Build history of the part. All positions in model axes, mm. A direction names the side the tool comes from. Coordinates: 2 decimals unless noted, no trailing zeros. Write each loop counter-clockwise with the first axis right and the second up, starting at its lowest first coordinate (ties: lowest second). Pieces come first, ordered by that corner, then holes.
```python
from build123d import *

# Parameters (mm, degrees)
SKETCH_1_W          = 37
SKETCH_1_H          = 37
EXTRUDE_1_DEPTH     = 11
SKETCH_2_R          = 1.5
CUT_EXTRUDE_1_DEPTH = 4
SKETCH_3_R          = 5.5
CUT_EXTRUDE_2_DEPTH = 29.381331893
SKETCH_4_R          = 7.5
CUT_EXTRUDE_4_DEPTH = 8
SKETCH_5_R          = 0.75
CUT_EXTRUDE_5_DEPTH = 28.358728041
SKETCH_7_W          = 8.873163899
SKETCH_7_H          = 2
SKETCH_7_W_2        = 8.897226177
SKETCH_7_W_3        = 2
SKETCH_7_H_2        = 11.172985464
EXTRUDE_3_DEPTH     = 5
EXTRUDE_6_DEPTH     = 8
EXTRUDE_7_REACH     = 44.805
EXTRUDE_8_REACH     = 44.805
CHAMFER_2_SIZE      = 3
SKETCH_11_R         = 0.75
CUT_EXTRUDE_6_DEPTH = 28.358728041
CHAMFER_3_SIZE      = 3
CHAMFER_3_SIZE2     = 4
FILLET_1_R          = 1
FILLET_2_R          = 1


with BuildPart() as part:
    # 草图1 → 凸台-拉伸1 (new body)
    with BuildSketch(Plane(origin=(0, 0, 0), x_dir=(1, 0, 0), z_dir=(0, 1, 0))):
        Rectangle(SKETCH_1_W, SKETCH_1_H)
    extrude(amount=EXTRUDE_1_DEPTH)

    # 草图2 → 切除-拉伸1 (cut)
    with BuildSketch(Plane.XZ):
        with Locations(Location((-16, 16, 0), (0, 0, 270))):
            Circle(SKETCH_2_R)
        with Locations(Location((-16, -16, 0), (0, 0, 270))):
            Circle(SKETCH_2_R)
        with Locations(Location((16, 16, 0), (0, 0, 270))):
            Circle(SKETCH_2_R)
        with Locations(Location((16, -16, 0), (0, 0, 270))):
            Circle(SKETCH_2_R)
        with Locations(Location((16, 4, 0), (0, 0, 270))):
            Circle(SKETCH_2_R)
        with Locations(Location((-16, 4, 0), (0, 0, 270))):
            Circle(SKETCH_2_R)
        with Locations(Location((0, 16, 0), (0, 0, 270))):
            Circle(SKETCH_2_R)
    extrude(amount=-CUT_EXTRUDE_1_DEPTH, mode=Mode.SUBTRACT)

    # 草图3 → 切除-拉伸2 (cut, through all)
    with BuildSketch(Plane.XZ):
        with Locations(Location((0, 0, 0), (0, 0, 270))):
            Circle(SKETCH_3_R)
    extrude(amount=-CUT_EXTRUDE_2_DEPTH, mode=Mode.SUBTRACT)

    # 草图4 → 切除-拉伸4 (cut)
    with BuildSketch(Plane.XZ):
        with BuildLine():
            Line((-16.5, 0.535898385), (-16.5, -12.535898385))
            ThreePointArc((-16.5, -12.535898385), (-13.525126266, -13.525126266), (-12.535898385, -16.5))
            Line((-12.535898385, -16.5), (12.535898385, -16.5))
            ThreePointArc((12.535898385, -16.5), (13.525126266, -13.525126266), (16.5, -12.535898385))
            Line((16.5, -12.535898385), (16.5, 0.535898385))
            ThreePointArc((16.5, 0.535898385), (12.5, 4), (16.5, 7.464101615))
            Line((16.5, 7.464101615), (16.5, 12.535898385))
            ThreePointArc((16.5, 12.535898385), (13.525126266, 13.525126266), (12.535898385, 16.5))
            Line((12.535898385, 16.5), (3.464101615, 16.5))
            ThreePointArc((3.464101615, 16.5), (0, 12.5), (-3.464101615, 16.5))
            Line((-3.464101615, 16.5), (-12.535898385, 16.5))
            ThreePointArc((-12.535898385, 16.5), (-13.525126266, 13.525126266), (-16.5, 12.535898385))
            Line((-16.5, 12.535898385), (-16.5, 7.464101615))
            ThreePointArc((-16.5, 7.464101615), (-12.5, 4), (-16.5, 0.535898385))
        make_face()
        with Locations(Location((0, 0, 0), (0, 0, 270))):
            Circle(SKETCH_4_R, mode=Mode.SUBTRACT)
    extrude(amount=-CUT_EXTRUDE_4_DEPTH, mode=Mode.SUBTRACT)

    # 草图5 → 切除-拉伸5 (cut, through all)
    with BuildSketch(Plane.XZ.offset(-8)):
        with Locations(Location((-8, 14, 0), (0, 0, 270))):
            Circle(SKETCH_5_R)
        with Locations(Location((0, 10.5, 0), (0, 0, 270))):
            Circle(SKETCH_5_R)
        with Locations(Location((8, 14, 0), (0, 0, 270))):
            Circle(SKETCH_5_R)
    extrude(amount=-CUT_EXTRUDE_5_DEPTH, mode=Mode.SUBTRACT)

    # 草图7 → 凸台-拉伸3 (add)
    with BuildSketch(Plane.XZ.offset(-8)):
        with Locations((-9.263191889, 4)):
            Rectangle(SKETCH_7_W, SKETCH_7_H)
        with Locations((9.460856753, 4)):
            Rectangle(SKETCH_7_W_2, SKETCH_7_H)
        with Locations((0, -11.893119293)):
            Rectangle(SKETCH_7_W_3, SKETCH_7_H_2)
    extrude(amount=EXTRUDE_3_DEPTH)

    # 草图6 → 凸台-拉伸6 (add)
    with BuildSketch(Plane.XZ.offset(-8)):
        Polygon((-11, 12.75), (-3.5, 12.75), (3.5, 12.75), (11, 12.75), (11, 17.612391956), (12, 17.612391956), (12, 11.75), (4.5, 11.75), (4.5, 5.286247788), (3.5, 5.286247788), (3.5, 11.75), (-3.5, 11.75), (-3.5, 5.286247788), (-4.5, 5.286247788), (-4.5, 11.75), (-12, 11.75), (-12, 17.612391956), (-11, 17.612391956), align=None)
    extrude(amount=EXTRUDE_6_DEPTH)

    # 凸台-拉伸7: up to this face of the body (flat: up to its plane)
    extrude_7_end = Plane(part.part.faces().sort_by_distance((0, 5.5, -18.5))[0])
    # 草图9 → 凸台-拉伸7 (add, up to the picked face)
    with BuildSketch(Plane.XY.offset(18.5), mode=Mode.PRIVATE) as extrude_7_sk1:
        Polygon((-12.5, 11), (-18.5, 5), (-18.5, 11), align=None)
    extrude_7_tool1 = split(extrude(extrude_7_sk1.sketch, amount=-EXTRUDE_7_REACH, mode=Mode.PRIVATE), bisect_by=extrude_7_end, keep=Keep.BOTH, mode=Mode.PRIVATE)
    # 草图9 → 凸台-拉伸7 (add, up to the picked face)
    with BuildSketch(Plane.XY.offset(18.5), mode=Mode.PRIVATE) as extrude_7_sk2:
        Polygon((18.5, 11), (12.5, 11), (18.5, 5), align=None)
    extrude_7_tool2 = split(extrude(extrude_7_sk2.sketch, amount=-EXTRUDE_7_REACH, mode=Mode.PRIVATE), bisect_by=extrude_7_end, keep=Keep.BOTH, mode=Mode.PRIVATE)
    add(extrude_7_tool1.solids().sort_by(Axis((-16.5, 9, 18.5), (0, 0, -1)))[0])
    add(extrude_7_tool2.solids().sort_by(Axis((16.5, 9, 18.5), (0, 0, -1)))[0])

    # 凸台-拉伸8: up to this face of the body (flat: up to its plane)
    extrude_8_end = Plane(part.part.faces().sort_by_distance((18.5, 5.5, 0))[0])
    # 草图10 → 凸台-拉伸8 (add, up to the picked face)
    with BuildSketch(Plane.ZY.offset(18.5), mode=Mode.PRIVATE) as extrude_8_sk1:
        Polygon((-12.5, 11), (-18.5, 5), (-18.5, 11), align=None)
    extrude_8_tool1 = split(extrude(extrude_8_sk1.sketch, amount=-EXTRUDE_8_REACH, mode=Mode.PRIVATE), bisect_by=extrude_8_end, keep=Keep.BOTH, mode=Mode.PRIVATE)
    # 草图10 → 凸台-拉伸8 (add, up to the picked face)
    with BuildSketch(Plane.ZY.offset(18.5), mode=Mode.PRIVATE) as extrude_8_sk2:
        Polygon((18.5, 11), (12.5, 11), (18.5, 5), align=None)
    extrude_8_tool2 = split(extrude(extrude_8_sk2.sketch, amount=-EXTRUDE_8_REACH, mode=Mode.PRIVATE), bisect_by=extrude_8_end, keep=Keep.BOTH, mode=Mode.PRIVATE)
    add(extrude_8_tool1.solids().sort_by(Axis((-18.5, 9, -16.5), (1, 0, 0)))[0])
    add(extrude_8_tool2.solids().sort_by(Axis((-18.5, 9, 16.5), (1, 0, 0)))[0])

    # 倒角2
    chamfer_2_edges = [part.edges().sort_by_distance(p)[0] for p in [
        (-18.5, 11, 0),
        (0, 11, 18.5),
        (18.5, 11, 0),
        (0, 11, -18.5),
    ]]
    chamfer(chamfer_2_edges, length=CHAMFER_2_SIZE)

    # 草图11 → 切除-拉伸6 (cut, through all)
    with BuildSketch(Plane.XZ.offset(-8)):
        with Locations(Location((8, 14, 0), (0, 0, 270))):
            Circle(SKETCH_11_R)
        with Locations(Location((-8, 14, 0), (0, 0, 270))):
            Circle(SKETCH_11_R)
    extrude(amount=-CUT_EXTRUDE_6_DEPTH, mode=Mode.SUBTRACT)

    # 倒角3
    chamfer_3_edges = [part.edges().sort_by_distance(p)[0] for p in [
        (0, 11, 5.5),
    ]]
    chamfer_3_side = [part.faces().sort_by_distance(p)[0] for p in [
        (0, 5.5, 5.5),
    ]]
    chamfer(chamfer_3_edges, length=CHAMFER_3_SIZE, length2=CHAMFER_3_SIZE2, reference=chamfer_3_side[0])

    # 圆角1
    # the kernel refuses this fillet: 1 mm, written as the material it takes off along each edge
    with BuildSketch(Plane(origin=(0, 11, 0), x_dir=(0, 0, -1), z_dir=(-1, 0, 0))) as fillet_1_piece_1:
        with BuildLine():
            CenterArc((9.5 + FILLET_1_R * 0.333333333333, FILLET_1_R), FILLET_1_R, 233.130102354, 36.869897646)
            Line((9.5 - FILLET_1_R * 0.266666666667, FILLET_1_R * 0.2), (9.5, 0))
            Line((9.5, 0), (9.5 + FILLET_1_R * 0.333333333333, 0))
        make_face()
    revolve(axis=Axis((0, 11, 0), (0, -1, 0)), mode=Mode.SUBTRACT)

    # 圆角2
    fillet_2_edges = [part.edges().sort_by_distance(p)[0] for p in [
        (0, 8, 5.5),
    ]]
    fillet(fillet_2_edges, radius=FILLET_2_R)


solid = part.part
```
1. Saw through at B-B on y = 8.75. List the corners of the cut face in (x, z), plus the area to 3 significant figures.
Computed values:
outline: (-17.75, -17.75) - (17.75, -17.75) - (17.75, 17.75) - (-17.75, 17.75) - close; hole circle Ø1.5 at (-8, 14); hole circle Ø13 at (0, 0); hole circle Ø1.5 at (0, 10.5); hole circle Ø1.5 at (8, 14)
area: 1,120 mm2
2. 3-axis set-ups, long thin cutter, end or side, ignore diameter. For faces 3 (the face through (0.03, 9.48, 11.25)), 4 (the face through (16, 7.5, -5.9)): which of +Z, -Z, +X, -X, +Y, -Y reach the whole face in a straight line?
Computed values:
face 3: +Y, -Y
face 4: -Y
3. Mould opens along Z. For faces 1 (the face through (17, 9.5, 0.3)), 2 (the face through (12.3, 7.5, 16)) say: +Z half, -Z half, draft (parallel to the pull), parting line (faces both ways), or undercut.
Computed values:
face 1: draft
face 2: undercut
4. Saw through at A-A on z = 10.5. List the corners of the cut face in (x, y), plus the area to 4 significant figures.
Computed values:
outline: (-18.5, 0) - (-16.5, 0) - (-16.5, 7) - (-15.5, 8) - (-4.5, 8) - (-4.5, 0) - (-3.5, 0) - (-3.5, 8) - (-0.75, 8) - (-0.75, 11) - (-15.5, 11) - (-18.5, 8) - close; (0.75, 8) - (3.5, 8) - (3.5, 0) - (4.5, 0) - (4.5, 8) - (15.5, 8) - (16.5, 7) - (16.5, 0) - (18.5, 0) - (18.5, 8) - (15.5, 11) - (0.75, 11) - close
area: 146.5 mm2
5. Flat gauge pins, fed straight in: pin 1 (2.5 mm diameter, centred on x = 16, z = 16, fed in from -Y); pin 2 (3 mm diameter, centred on y = 10, z = 1, fed in from -X); pin 3 (0.6 mm diameter, centred on x = 9, z = 4.5, fed in from -Y). Where does each tip first touch, or does it go through?
Computed values:
pin 1: stops at y = 4
pin 2: stops at x = -18
pin 3: stops at y = 3
6. Saw through at C-C on x = -10.5. List the corners of the cut face in (y, z), plus the area to 3 significant figures.
Computed values:
outline: (0, -18.5) - (8, -18.5) - (11, -15.5) - (11, 15.5) - (8, 18.5) - (0, 18.5) - (0, 16.5) - (7, 16.5) - (8, 15.5) - (8, 12.75) - (0, 12.75) - (0, 11.75) - (8, 11.75) - (8, 5) - (3, 5) - (3, 3) - (8, 3) - (8, -15.5) - (7, -16.5) - (0, -16.5) - close
area: 153 mm2
7. Probe line 1 along X through (y, z) = (5, 12); line 2 along X through (y, z) = (6.5, 8.5); line 3 along Z through (x, y) = (-11.5, 7). List the from-to ranges inside material, lowest first.
Computed values:
line 1: x = -18.5 to -16.5, -12 to 12, 16.5 to 18.5
line 2: x = -18.5 to -16.5, -4.5 to -3.5, 3.5 to 4.5, 16.5 to 18.5
line 3: z = -18.5 to -16.5, 3 to 5, 11.75 to 18.5
